```python
from build123d import *

# Parameters (mm, degrees)
CROQUIS1_W              = 60
CROQUIS1_H              = 125
SALIENTE_EXTRUIR1_DEPTH = 20
CROQUIS2_R              = 4
CORTAR_EXTRUIR1_DEPTH   = 25
CORTAR_EXTRUIR2_START   = -25
CROQUIS3_R              = 4
CORTAR_EXTRUIR2_DEPTH   = 25


with BuildPart() as part:
    # Croquis1 → Saliente-Extruir1 (new body)
    with BuildSketch(Plane(origin=(0, 0, 0), x_dir=(0, 0, -1), z_dir=(1, 0, 0))):
        Rectangle(CROQUIS1_W, CROQUIS1_H)
    extrude(amount=SALIENTE_EXTRUIR1_DEPTH)

    # Croquis2 → Cortar-Extruir1 (cut)
    with BuildSketch(Plane(origin=(0, 62.5, 0), x_dir=(1, 0, 0), z_dir=(0, 1, 0))):
        with Locations(Location((10, 20, 0), (0, 0, 270))):
            Circle(CROQUIS2_R)
        with Locations(Location((10, -20, 0), (0, 0, 270))):
            Circle(CROQUIS2_R)
    extrude(amount=-CORTAR_EXTRUIR1_DEPTH, mode=Mode.SUBTRACT)

    # Croquis3 → Cortar-Extruir2 (cut)
    with BuildSketch(Plane.XZ.offset(62.5).offset(CORTAR_EXTRUIR2_START)):
        with Locations(Location((10, 20, 0), (0, 0, 90))):
            Circle(CROQUIS3_R)
        with Locations(Location((10, -20, 0), (0, 0, 90))):
            Circle(CROQUIS3_R)
    extrude(amount=CORTAR_EXTRUIR2_DEPTH, mode=Mode.SUBTRACT)


solid = part.part
```
Check sheet for the modelled part. Datum: model origin and axes. Units: mm. A direction names the side the tool comes from. Round coordinates to 2 decimals unless told otherwise and drop trailing zeros. Write each loop counter-clockwise with the first axis right and the second up, starting at its lowest first coordinate (ties: lowest second). Pieces come first, ordered by that corner, then holes. Notation, with made-up numbers: M -40,79.5 L -6,79.5 A18 ccw -6,97.5 Z; hole C 34.25,31.25 d1. An arc over 180 degrees is marked long. Write item = value, one per line. Start each with the question number.
1. Section check D-D, the plane z = -17.5. Record the cut outline in (x, y), then the cut area to 3 significant figures.
2. Gauge pin test, flat ends, axial feed: pin 1 (5 mm diameter, centred on x = 10, z = 20, fed in from +Y); pin 2 (4 mm diameter, centred on x = 9.5, z = 20, fed in from -Y). Record the tip position at first contact, or that the pin passes through.
3. Scan lines: line 1 (Z direction, x = 10, y = -42.5); line 2 (X direction, y = 55, z = 20); line 3 (Z direction, x = 13.25, y = 41.5). Record each from-to range of solid material in increasing order. Write a range as [from, to].
4. Section check A-A, the plane y = 43.5. Record the cut outline in (x, z).
5. Section check C-C, the plane x = 10. Record the cut outline in (y, z).
6. Release check for a two-part mould opening along Z. For faces 4 (the flat face through (10, -1, -30)), 5 (the flat face through (10, -37.5, 20)), 6 (the flat face through (0, 1, 0)) record: pulls with the +Z half, pulls with the -Z half, needs draft (parallel to the pull), parting line crosses it, or undercut.
7. Section check B-B, the plane z = 20. Record the cut outline in (x, y), then the cut area to 3 significant figures.
8. Tool access check on faces 1 (the flat face through (10, -1, 30)), 2 (the cylindrical face through (12.4, -49.8, -23.2)), 3 (the flat face through (10, 37.5, -20)). Record the directions out of +Z, -Z, +X, -X, +Y, -Y that give a thin tool (end or side, any length) a straight path to the whole face; none if there is none.
Results found:
q1.outline = M 0,-62.5 L 6.88,-62.5 L 6.88,-37.5 L 13.12,-37.5 L 13.12,-62.5 L 20,-62.5 L 20,62.5 L 13.12,62.5 L 13.12,37.5 L 6.88,37.5 L 6.88,62.5 L 0,62.5 Z
q1.area = 2,190 mm^2
q2.pin_1 = 37.5
q2.pin_2 = -37.5
q3.line_1 = [-30, -24], [-16, 16], [24, 30]
q3.line_2 = [0, 6], [14, 20]
q3.line_3 = [-30, -22.33], [-17.67, 17.67], [22.33, 30]
q4.outline = M 0,-30 L 20,-30 L 20,30 L 0,30 Z; hole C 10,-20 d8; hole C 10,20 d8
q5.outline = M -62.5,-30 L 62.5,-30 L 62.5,-24 L 37.5,-24 L 37.5,-16 L 62.5,-16 L 62.5,16 L 37.5,16 L 37.5,24 L 62.5,24 L 62.5,30 L -62.5,30 L -62.5,24 L -37.5,24 L -37.5,16 L -62.5,16 L -62.5,-16 L -37.5,-16 L -37.5,-24 L -62.5,-24 Z
q6.face_4 = pulls with the -Z half
q6.face_5 = undercut
q6.face_6 = needs draft
q7.outline = M 0,-62.5 L 6,-62.5 L 6,-37.5 L 14,-37.5 L 14,-62.5 L 20,-62.5 L 20,62.5 L 14,62.5 L 14,37.5 L 6,37.5 L 6,62.5 L 0,62.5 Z
q7.area = 2,100 mm^2
q8.face_1 = +Z, +X, -X, +Y, -Y
q8.face_2 = -Y
q8.face_3 = +Y
